```python
from build123d import *

# Parameters (mm, degrees)
SKETCH1_R           = 10
EXTRUDE1_DEPTH      = 35
FILLET1_R           = 10
FILLET_1_R          = 8
SKETCH2_W           = 7.672344266
SKETCH2_H           = 13.422166089
EXTRUDE2_DEPTH      = 20
SKETCH5_W           = 6.488658855
SKETCH5_H           = 20.959398048
EXTRUDE4_DEPTH      = 38.749172176
SKETCH7_W           = 24.373627343
SKETCH7_H           = 7.918162835
SKETCH7_H_2         = 6.543162835
EXTRUDE6_DEPTH      = 46
SKETCH10_R          = 1.5
CUT_EXTRUDE2_DEPTH  = 37.464237757
CUT_EXTRUDE3_DEPTH  = 37.954575301
FILLET2_START       = -3
FILLET2_OUTLINE_R   = 1.5
FILLET2_DEPTH       = 6
FILLET3_R           = 20
CUT_EXTRUDE_1_DEPTH = 37.954575301
FILLET_2_R          = 10


with BuildPart() as part:
    # Sketch1 → Extrude1 (new body)
    with BuildSketch(Plane(origin=(0, 0, 0), x_dir=(1, 0, 0), z_dir=(0, 1, 0))):
        with Locations(Location((0, 0, 0), (0, 0, 270))):
            Circle(SKETCH1_R)
    extrude(amount=EXTRUDE1_DEPTH)

    # Fillet1
    fillet1_edges = [part.edges().sort_by_distance(p)[0] for p in [
        (0, 0, -10),
    ]]
    fillet(fillet1_edges, radius=FILLET1_R)

    # Скругление1
    fillet_1_edges = [part.edges().sort_by_distance(p)[0] for p in [
        (0, 35, -10),
    ]]
    fillet(fillet_1_edges, radius=FILLET_1_R)

    # Sketch2 → Extrude2 (cut, symmetric)
    with BuildSketch(Plane.XY):
        with Locations((6.836172133, 1.953557325)):
            Rectangle(SKETCH2_W, SKETCH2_H)
        with Locations((-6.836172133, 1.953557325)):
            Rectangle(SKETCH2_W, SKETCH2_H)
    extrude(amount=EXTRUDE2_DEPTH, both=True, mode=Mode.SUBTRACT)

    # Sketch5 → Extrude4 (cut, through all)
    with BuildSketch(Plane(origin=(0, 0, 0), x_dir=(1, 0, 0), z_dir=(0, 1, 0))):
        with Locations((8.244329428, 0.450601309)):
            Rectangle(SKETCH5_W, SKETCH5_H)
        with Locations((-8.244329428, 0.450601309)):
            Rectangle(SKETCH5_W, SKETCH5_H)
    extrude(amount=EXTRUDE4_DEPTH, mode=Mode.SUBTRACT)

    # Sketch7 → Extrude6 (cut, symmetric)
    with BuildSketch(Plane(origin=(0, 0, 0), x_dir=(1, 0, 0), z_dir=(0, 1, 0))):
        with Locations((-0.125613483, -8.959081418)):
            Rectangle(SKETCH7_W, SKETCH7_H)
        with Locations((-0.125613483, 9.646581418)):
            Rectangle(SKETCH7_W, SKETCH7_H_2)
    extrude(amount=EXTRUDE6_DEPTH, both=True, mode=Mode.SUBTRACT)

    # Sketch10 → Cut-Extrude2 (cut, through all)
    with BuildSketch(Plane(origin=(3, 0, 0), x_dir=(0, 0, -1), z_dir=(1, 0, 0))):
        with Locations(Location((3.202782465, 3.918341245, 0), (0, 0, 90))):
            Circle(SKETCH10_R)
    extrude(amount=-CUT_EXTRUDE2_DEPTH, mode=Mode.SUBTRACT)

    # Sketch12 → Cut-Extrude3 (cut, through all)
    with BuildSketch(Plane(origin=(5, 0, 0), x_dir=(0, 0, -1), z_dir=(1, 0, 0))):
        Polygon((-5, 15.421884283), (2.380521482, 8.664640369), (-3.375305401, -2.43292564), (-5, -2.43292564), align=None)
    extrude(amount=-CUT_EXTRUDE3_DEPTH, mode=Mode.SUBTRACT)

    # Fillet2: read off the stored shape, not the designer's step
    # Fillet2 outline → Fillet2 (add)
    with BuildSketch(Plane.YZ.offset(FILLET2_START)):
        with BuildLine():
            ThreePointArc((0.62964824, 1.787878044), (0.810500421, -2.559901853), (2.903566036, -6.375))
            Line((2.903566036, -6.375), (8.664640369, -6.375))
            Line((8.664640369, -6.375), (8.664640369, -2.380521482))
            Line((8.664640369, -2.380521482), (14.875593683, 4.403320413))
            ThreePointArc((14.875593683, 4.403320413), (8.191715719, 0.703912056), (0.62964824, 1.787878044))
        make_face()
        with Locations((3.918341245, -3.202782465)):
            Circle(FILLET2_OUTLINE_R, mode=Mode.SUBTRACT)
    extrude(amount=FILLET2_DEPTH)

    # Fillet3
    # the kernel refuses this fillet: 20 mm, written as the material it takes off along each edge
    with BuildSketch(Plane(origin=(14.71184435, 8.664640369, -2.380521482), x_dir=(0, 0.6752773616828561, 0.7375638852320802), z_dir=(-1, 0, 0))) as fillet3_piece_1_section:
        with BuildLine():
            CenterArc((7.08473774, 20), FILLET3_R, 239.897661879, 30.102338121)
            Line((-2.946183095, 2.697380915), (-3.146801512, 2.351328533))
            ThreePointArc((-3.146801512, 2.351328533), (-1.743202492, 1.053664903), (-0.270110945, -0.295025554))
            Line((-0.270110945, -0.295025554), (0, -0.4))
            Line((0, -0.4), (7.08473774, -0.4))
            Line((7.08473774, -0.4), (7.08473774, 0))
        make_face()
    fillet3_piece_1 = extrude(amount=37.423688699, mode=Mode.PRIVATE)
    fillet3_piece_1 = split(fillet3_piece_1, bisect_by=Plane(origin=(3, 8.664640369, -2.380521482), z_dir=(1, 0, 0)), keep=Keep.TOP, mode=Mode.PRIVATE)
    add(fillet3_piece_1, mode=Mode.SUBTRACT)
    with BuildSketch(Plane(origin=(-3, 8.664640369, -2.380521482), x_dir=(0, 0.6752773616828561, 0.7375638852320802), z_dir=(-1, 0, 0)), Plane(origin=(22.71184435, 8.664640369, -2.380521482), x_dir=(0, 0.6752773616828562, 0.7375638852320802), z_dir=(-1, 0, 0))) as fillet3_piece_2:
        with BuildLine():
            CenterArc((7.08473774, 20), FILLET3_R, 239.897661879, 30.102338121)
            Line((-2.946183095, 2.697380915), (-3.146801512, 2.351328533))
            ThreePointArc((-3.146801512, 2.351328533), (-1.743202492, 1.053664903), (-0.270110945, -0.295025554))
            Line((-0.270110945, -0.295025554), (0, -0.4))
            Line((0, -0.4), (7.08473774, -0.4))
            Line((7.08473774, -0.4), (7.08473774, 0))
        make_face()
    extrude(amount=19.71184435, mode=Mode.SUBTRACT)
    with BuildSketch(Plane(origin=(22.71184435, 8.664640369, -2.380521482), x_dir=(0, 0.6752773616828562, 0.7375638852320802), z_dir=(-1, 0, 0))) as fillet3_piece_3_section:
        with BuildLine():
            CenterArc((7.08473774, 20), FILLET3_R, 239.897661879, 30.102338121)
            Line((-2.946183095, 2.697380915), (-3.146801512, 2.351328533))
            ThreePointArc((-3.146801512, 2.351328533), (-1.743202492, 1.053664903), (-0.270110945, -0.295025554))
            Line((-0.270110945, -0.295025554), (0, -0.4))
            Line((0, -0.4), (7.08473774, -0.4))
            Line((7.08473774, -0.4), (7.08473774, 0))
        make_face()
    fillet3_piece_3 = extrude(amount=37.423688699, mode=Mode.PRIVATE)
    fillet3_piece_3 = split(fillet3_piece_3, bisect_by=Plane(origin=(-3, 8.664640369, -2.380521482), z_dir=(-1, 0, 0)), keep=Keep.TOP, mode=Mode.PRIVATE)
    add(fillet3_piece_3, mode=Mode.SUBTRACT)

    # Эскиз1 → Вырез-Вытянуть1 (cut, through all)
    with BuildSketch(Plane(origin=(5, 0, 0), x_dir=(0, 0, -1), z_dir=(1, 0, 0))):
        Polygon((-4.197009704, 35.90598138), (7.773675874, 35.90598138), (7.773675874, 14.167506287), align=None)
    extrude(amount=-CUT_EXTRUDE_1_DEPTH, mode=Mode.SUBTRACT)

    # Скругление2
    fillet_2_edges = [part.edges().sort_by_distance(p)[0] for p in [
        (-1.1e-08, 16.707467799, -6.375),
    ]]
    fillet(fillet_2_edges, radius=FILLET_2_R)


solid = part.part
```
Verification items for the finished model (mm, model axes). A direction names the side the tool comes from. Round coordinates to 2 decimals unless told otherwise and drop trailing zeros. Order: outer loops, then holes, each group sorted by start corner. A loop starts at its lowest first (then second) coordinate and runs counter-clockwise, first axis right, second up.
1) Material ranges on line 1 (X direction, y = 3.5, z = -1); line 2 (Y direction, x = -0.5, z = -2); line 3 (Z direction, x = -1.75, y = 9) (3 decimals), recorded low to high.
Geometry says:
line 1: x = -3 to 3
line 2: y = 0.21 to 3.02, 4.81 to 24.65
line 3: z = -6.375 to 0.881
2) Tool access check on faces 4 (the flat face through (-5, 18, 1)), 5 (the flat face through (5, 18, 1)), 6 (the flat face through (-3, 6, -2)), 7 (the flat face through (0.07, 15.11, 4.66)), 8 (the flat face through (3, 6, -2)). Record the directions out of +Z, -Z, +X, -X, +Y, -Y that give a thin tool (end or side, any length) a straight path to the whole face; none if there is none.
Geometry says:
face 4: +Z, -Z, -X, +Y, -Y
face 5: +Z, -Z, +X, +Y, -Y
face 6: +Z, -X, -Y
face 7: +Z, -Y
face 8: +Z, +X, -Y
3) Cross-section at A-A, the plane y = 11.5. Record the cut outline in (x, z) (3 decimals), plus the area to 3 significant figures.
Geometry says:
outline: (-5, -6.375) - (5, -6.375) - (5, 0.344) - (3, 0.344) - (3, 1.829) - (-3, 1.829) - (-3, 0.344) - (-5, 0.344) - close
area: 76.1 mm2
4) Cross-section at C-C, the plane y = 17. Record the cut outline in (x, z).
Geometry says:
outline: (-5, -5.96) - (5, -5.96) - (5, 5) - (-5, 5) - close
5) Draft check along Y on faces 1 (the flat face through (0.07, 26.787, -0.824)), 2 (the cylindrical face through (-0.042, 8.299, 0.724)), 3 (the cylindrical face through (4.014, 10.414, -1.514)). Enter one of: +Y half, -Y half, draft (parallel to the pull), parting line (faces both ways), or undercut.
Geometry says:
face 1: +Y half
face 2: undercut
face 3: -Y half
6) Depth check by flat-ended pin: pin 1 (1.5 mm diameter, centred on x = -4, z = -1.5, fed in from +Y); pin 2 (1 mm diameter, centred on x = 2, z = 3, fed in from -Y). Enter the tip coordinate at first touch or a pass-through.
Geometry says:
pin 1: stops at y = 26.92
pin 2: stops at y = 12.65
7) Cross-section at B-B, the plane y = 24. Record the cut outline in (x, z), plus the area to 3 significant figures.
Geometry says:
outline: (-5, -2.36) - (5, -2.36) - (5, 5) - (-5, 5) - close
area: 73.6 mm2
